Design review of the part shown in the three views and the two pictorial views. Dimensions are in mm from the part's minimum x, y and z. Give positions to 0.01 mm unless a question says otherwise; leave off trailing zeros. Order: outer loops, then holes, each group sorted by start corner. A loop starts at its lowest first (then second) coordinate and runs counter-clockwise, first axis right, second up.
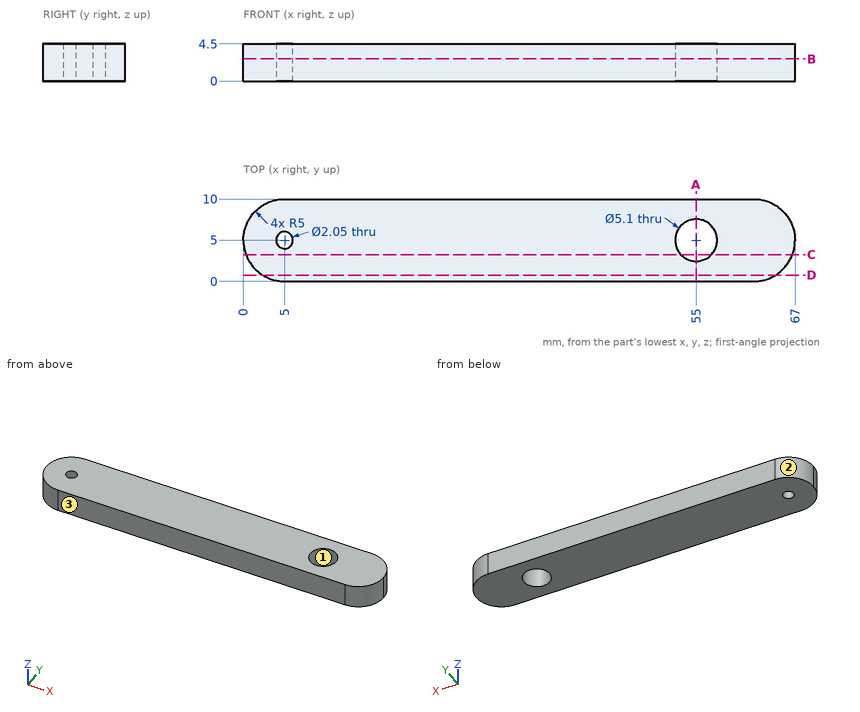
1) Clearance check with flat-ended pins moving along their axes: pin 1 (2 mm diameter, centred on x = 8.5, y = 8, fed in from -Z); pin 2 (1 mm diameter, centred on y = 1.5, z = 3.5, fed in from -X). State where each tip first meets the part, or that it passes through.
Answer sheet:
pin 1: stops at z = 0
pin 2: stops at x = 1
2) We need section D-D on y = 0.75. Give the boundary of the cut face in (x, z).
Answer sheet:
outline: (2.37, 0) - (64.63, 0) - (64.63, 4.5) - (2.37, 4.5) - close
3) We need section B-B on z = 2.7. Count the separate pieces of the cut face and the enclosed holes in it, then the cut area to 3 significant figures.
Answer sheet:
separate pieces: 1
enclosed holes: 2
area: 625 mm2
4) We need section A-A on x = 55. Give the boundary of the cut face in (y, z).
Answer sheet:
outline: (0, 0) - (2.45, 0) - (2.45, 4.5) - (0, 4.5) - close; (7.55, 0) - (10, 0) - (10, 4.5) - (7.55, 4.5) - close
5) We need section C-C on y = 3.25. Give the boundary of the cut face in (x, z).
Answer sheet:
outline: (0.32, 0) - (53.15, 0) - (53.15, 4.5) - (0.32, 4.5) - close; (56.85, 0) - (66.68, 0) - (66.68, 4.5) - (56.85, 4.5) - close
6) To check wall thickness, follow line 1 (Y direction, x = 55, z = 1.2); line 2 (Y direction, x = 5, z = 2.7) (3 decimals); line 3 (X direction, y = 4.75, z = 0.5). State the ranges of each line that lie inside material, in increasing order.
Answer sheet:
line 1: y = 0 to 2.45, 7.55 to 10
line 2: y = 0 to 3.975, 6.025 to 10
line 3: x = 0.01 to 4.01, 5.99 to 52.46, 57.54 to 66.99
7) Draft analysis for pull direction X (two halves, no side actions). For the marked faces 1, 2 and 3, state which applies: +X half, -X half, draft (parallel to the pull), parting line (faces both ways), or undercut.
Answer sheet:
face 1: undercut
face 2: -X half
face 3: draft
